Part print with two shaded views. Sizes in mm from the minimum x, y, z corner. Round coordinates to 2 decimals unless told otherwise and drop trailing zeros. Write each loop counter-clockwise with the first axis right and the second up, starting at its lowest first coordinate (ties: lowest second). Pieces come first, ordered by that corner, then holes. Notation, with made-up numbers: (72.25, 49.25) - (118.25, 49.25) arc R21 cw to (118.25, 68.25) - close; hole circle Ø3 at (57.25, -6.5). An arc over 180 degrees is marked (long way). Answer as a JSON object with one key per item and string values. Group by question number.
Item 1: Probe line 1 (Y direction, x = 30, z = 23.9); line 2 (Z direction, x = 5.5, y = 45.5); line 3 (Z direction, x = 25, y = 45). List the from-to ranges inside material, lowest first. Write a range as from..to.
Item 2: Two-plate mould, pull along Y, no slides. Class the marked faces 1, 2 and 3: +Y half, -Y half, draft (parallel to the pull), parting line (faces both ways), or undercut.
Item 3: Slice it at C-C, the plane z = 3. List the corners of the cut face in (x, y).
Item 4: Slice it at D-D, the plane x = 5. List the corners of the cut face in (y, z), then the cut area to 3 significant figures.
Item 5: Flat gauge pins, fed straight in: pin 1 (4 mm diameter, centred on x = 51, z = 21, fed in from +Y) (1 decimal); pin 2 (12 mm diameter, centred on x = 36, z = 20, fed in from -Y); pin 3 (5 mm diameter, centred on y = 14.5, z = 10.5, fed in from +X) (1 decimal); pin 4 (4.5 mm diameter, centred on x = 9.85, y = 50.15, fed in from -Z). Where does each tip first touch, or does it go through?
Item 6: Slice it at A-A, the plane y = 30. List the corners of the cut face in (x, z).
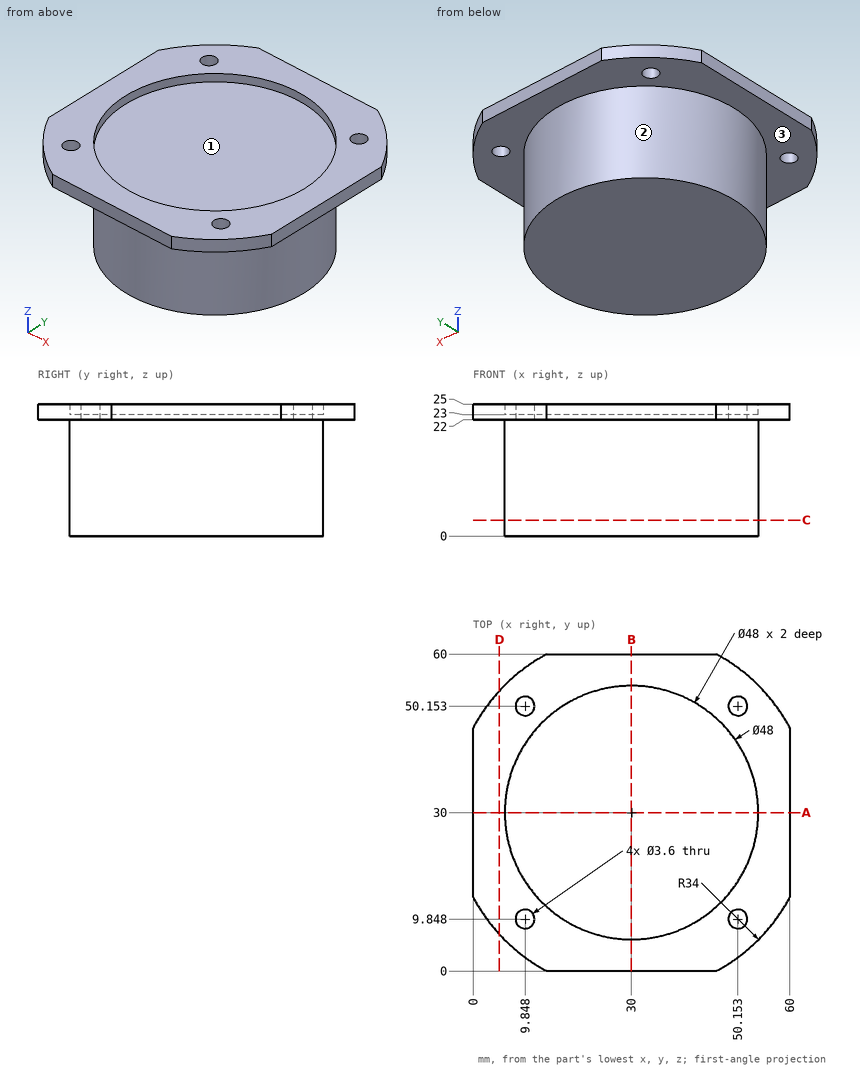
Geometry says:
{
 "1": {"line 1": "y = 0..6, 54..60", "line 2": "z = 22..25", "line 3": "z = 0..23"},
 "2": {"face 1": "undercut", "face 2": "parting line", "face 3": "draft"},
 "3": {"outline": "circle Ø48 at (30, 30)"},
 "4": {"outline": "(6.96, 22) - (53.04, 22) - (53.04, 25) - (6.96, 25) - close", "area": "138 mm^2"},
 "5": {"pin 1": "stops at y = 58", "pin 2": "stops at y = 0", "pin 3": "stops at x = 50.2", "pin 4": "stops at z = 22"},
 "6": {"outline": "(0, 22) - (6, 22) - (6, 0) - (54, 0) - (54, 22) - (60, 22) - (60, 25) - (54, 25) - (54, 23) - (6, 23) - (6, 25) - (0, 25) - close"}
}
